from build123d import *
from build123d.topology import SkipClean

# Parameters (mm, degrees)
CROQUIS3_W                   = 38
CROQUIS3_H                   = 38
SALIENTE_EXTRUIR9_DEPTH      = 1
SALIENTE_EXTRUIR10_START     = -11
SALIENTE_EXTRUIR10_OUTLINE_W = 38
SALIENTE_EXTRUIR10_OUTLINE_H = 38
SALIENTE_EXTRUIR10_DEPTH     = 10
CROQUIS13_W                  = 38
CROQUIS13_H                  = 38
SALIENTE_EXTRUIR15_DEPTH     = 3
CROQUIS14_R                  = 1.5
CORTAR_EXTRUIR1_DEPTH        = 14
CROQUIS15_W                  = 38
CROQUIS15_H                  = 24.129942315
CROQUIS15_R                  = 1.5
CROQUIS15_R_2                = 3.5
SALIENTE_EXTRUIR16_DEPTH     = 1
CORTAR_EXTRUIR2_DEPTH        = 14
CROQUIS17_R                  = 1.5
SALIENTE_EXTRUIR17_DEPTH     = 5
CROQUIS18_R                  = 1.5
CROQUIS18_W                  = 12
CROQUIS18_H                  = 12
SALIENTE_EXTRUIR18_DEPTH     = 5
CORTAR_EXTRUIR3_DEPTH        = 3
CROQUIS20_R                  = 3
CROQUIS20_R_2                = 1.5
SALIENTE_EXTRUIR19_DEPTH     = 3
REDONDEO11_R                 = 1
CROQUIS21_W                  = 12
CROQUIS21_H                  = 3
SALIENTE_EXTRUIR20_DEPTH     = 10


# Read off the part's stored shape, not the designer's step: Saliente-Extruir10
with BuildPart() as part:
    # Croquis3 → Saliente-Extruir9 (new body)
    with BuildSketch(Plane.XY.offset(5)):
        Polygon((19, -5.370057685), (26.870057685, 2.5), (26.870057685, 40.5), (19, 48.370057685), (-19, 48.370057685), (-26.870057685, 40.5), (-26.870057685, 2.5), (-19, -5.370057685), align=None)
        with Locations((0, 21.5)):
            Rectangle(CROQUIS3_W, CROQUIS3_H, mode=Mode.SUBTRACT)
    extrude(amount=-SALIENTE_EXTRUIR9_DEPTH)

    # Saliente-Extruir10 outline → Saliente-Extruir10 (add)
    with BuildSketch(Plane(origin=(0, 0, 4), x_dir=(-1, 0, 0), z_dir=(0, 0, -1)).offset(SALIENTE_EXTRUIR10_START)):
        Polygon((-26.870057685, 2.5), (-19, -5.370057685), (19, -5.370057685), (26.870057685, 2.5), (26.870057685, 40.5), (19, 48.370057685), (-19, 48.370057685), (-26.870057685, 40.5), align=None)
        with Locations((0, 21.5)):
            Rectangle(SALIENTE_EXTRUIR10_OUTLINE_W, SALIENTE_EXTRUIR10_OUTLINE_H, mode=Mode.SUBTRACT)
    extrude(amount=SALIENTE_EXTRUIR10_DEPTH)

    # Croquis13 → Saliente-Extruir15 (add)
    with BuildSketch(Plane.XY.offset(15)):
        with BuildLine():
            Line((-22.5, 44.870057685), (-22.5, -1))
            Line((-22.5, -1), (22.5, -1))
            Line((22.5, -1), (22.5, 44.870057685))
            Line((22.5, 44.870057685), (19.292893219, 48.077164466))
            ThreePointArc((19.292893219, 48.077164466), (18.96846987, 48.293937218), (18.585786438, 48.370057685))
            Line((18.585786438, 48.370057685), (-18.585786438, 48.370057685))
            ThreePointArc((-18.585786438, 48.370057685), (-18.96846987, 48.293937218), (-19.292893219, 48.077164466))
            Line((-19.292893219, 48.077164466), (-22.5, 44.870057685))
        make_face()
        with Locations((0, 21.5)):
            Rectangle(CROQUIS13_W, CROQUIS13_H, mode=Mode.SUBTRACT)
    extrude(amount=SALIENTE_EXTRUIR15_DEPTH)

    # Croquis14 → Cortar-Extruir1 (cut)
    with BuildSketch(Plane(origin=(0, 0, 4), x_dir=(-1, 0, 0), z_dir=(0, 0, -1))):
        with Locations((10, 44.97415474)):
            Circle(CROQUIS14_R)
        with Locations(Location((-10, 44.97415474, 0), (0, 0, 180))):
            Circle(CROQUIS14_R)
    extrude(amount=-CORTAR_EXTRUIR1_DEPTH, mode=Mode.SUBTRACT)

    # Croquis15 → Saliente-Extruir16 (add)
    with BuildSketch(Plane(origin=(0, 0, 4), x_dir=(-1, 0, 0), z_dir=(0, 0, -1))):
        with Locations((0, 28.435028843)):
            Rectangle(CROQUIS15_W, CROQUIS15_H)
        with Locations((0, 34.97415474)):
            Circle(CROQUIS15_R, mode=Mode.SUBTRACT)
        with Locations((0, 25.370057685)):
            Circle(CROQUIS15_R_2, mode=Mode.SUBTRACT)
    extrude(amount=-SALIENTE_EXTRUIR16_DEPTH)

    # Croquis16 → Cortar-Extruir2 (cut)
    with BuildSketch(Plane(origin=(0, 0, 4), x_dir=(-1, 0, 0), z_dir=(0, 0, -1))):
        Polygon((-19, 2.5), (-19, 16.370057685), (-26.870057685, 24.24011537), (-26.870057685, 2.5), (-19, -5.370057685), (19, -5.370057685), (26.870057685, 2.5), (26.870057685, 24.24011537), (19, 16.370057685), (19, 2.5), align=None)
    extrude(amount=-CORTAR_EXTRUIR2_DEPTH, mode=Mode.SUBTRACT)

    # Croquis17 → Saliente-Extruir17 (add)
    with SkipClean():  # the faces are left unmerged after this step: merging them gives an invalid solid
        with BuildSketch(Plane.XY.offset(5)):
            Polygon((6, 31.370057685), (6, 25.370057685), (6, 19.370057685), (6, 16.370057685), (19, 16.370057685), (19, 40.5), (-19, 40.5), (-19, 16.370057685), (-6, 16.370057685), (-6, 19.370057685), (-6, 31.370057685), align=None)
            with Locations((0, 34.97415474)):
                Circle(CROQUIS17_R, mode=Mode.SUBTRACT)
        extrude(amount=SALIENTE_EXTRUIR17_DEPTH)
    add(part.part.scale(1), mode=Mode.REPLACE)  # the faces are merged on a copy

    # Croquis18 → Saliente-Extruir18 (add)
    # profile 1 of 2: a face of its own
    with BuildSketch(Plane.XY.offset(10)):
        Polygon((-6, 31.370057685), (6, 31.370057685), (6, 16.370057685), (19, 16.370057685), (19, 40.5), (-19, 40.5), (-19, 16.370057685), (-6, 16.370057685), align=None)
        with Locations(Location((0, 34.97415474, 0), (0, 0, 180))):
            Circle(CROQUIS18_R, mode=Mode.SUBTRACT)
    # profile 2 of 2: a face of its own
    with BuildSketch(Plane.XY.offset(10)):
        with Locations((0, 25.370057685)):
            Rectangle(CROQUIS18_W, CROQUIS18_H)
    extrude(amount=SALIENTE_EXTRUIR18_DEPTH)

    # Croquis19 → Cortar-Extruir3 (cut)
    with BuildSketch(Plane.XY.offset(18)):
        Polygon((-22.5, 19.870057685), (-19, 16.370057685), (-19, 21.370057685), (-22.5, 21.370057685), align=None)
        Polygon((19, 16.370057685), (22.5, 19.870057685), (22.5, 21.370057685), (19, 21.370057685), align=None)
    extrude(amount=-CORTAR_EXTRUIR3_DEPTH, mode=Mode.SUBTRACT)

    # Croquis20 → Saliente-Extruir19 (add)
    with BuildSketch(Plane.XY.offset(15)):
        with Locations(Location((0, 34.97415474, 0), (0, 0, 180))):
            Circle(CROQUIS20_R)
        with Locations(Location((0, 34.97415474, 0), (0, 0, 180))):
            Circle(CROQUIS20_R_2, mode=Mode.SUBTRACT)
    extrude(amount=SALIENTE_EXTRUIR19_DEPTH)

    # Redondeo11
    redondeo11_edges = [part.edges().sort_by_distance(p)[0] for p in [
        (26.870057685, 40.5, 10),
        (19, 48.370057685, 10),
        (-19, 48.370057685, 10),
        (-26.870057685, 40.5, 10),
        (26.870057685, 24.24011537, 9.5),
        (19, 16.370057685, 9.5),
        (-26.870057685, 24.24011537, 9.5),
        (-19, 16.370057685, 9.5),
    ]]
    fillet(redondeo11_edges, radius=REDONDEO11_R)

    # Croquis21 → Saliente-Extruir20 (add)
    with BuildSketch(Plane.XY.offset(5)):
        with Locations((0, 17.870057685)):
            Rectangle(CROQUIS21_W, CROQUIS21_H)
    extrude(amount=SALIENTE_EXTRUIR20_DEPTH)


solid = part.part
Design review of the part built by this model. Coordinates are the model's own, in mm. A direction names the side the tool comes from. Give positions to 0.01 mm unless a question says otherwise; leave off trailing zeros. Order: outer loops, then holes, each group sorted by start corner. A loop starts at its lowest first (then second) coordinate and runs counter-clockwise, first axis right, second up.
1. Add section A-A, the plane z = 17.25. State the section outline as (x, y) points, then the cut area to 3 significant figures.
Solution:
outline: (-22.5, 21.37) - (-19, 21.37) - (-19, 40.5) - (19, 40.5) - (19, 21.37) - (22.5, 21.37) - (22.5, 44.87) - (19.29, 48.08) arc R1 ccw to (18.59, 48.37) - (-18.59, 48.37) arc R1 ccw to (-19.29, 48.08) - (-22.5, 44.87) - close; circle Ø6 at (0, 34.97); hole circle Ø3 at (-10, 44.97); hole circle Ø3 at (0, 34.97); hole circle Ø3 at (10, 44.97)
area: 483 mm2
2. To check wall thickness, follow L1, parallel to Y at x = 0, z = 4.65; L2, parallel to Y at x = -10, z = 8.25; L3, parallel to X at y = 25, z = 15.25. State the ranges of each line that lie inside material, in increasing order.
Solution:
L1: y = 16.37 to 21.87, 28.87 to 33.47, 36.47 to 48.37
L2: y = 16.37 to 43.47, 46.47 to 48.37
L3: x = -22.5 to -19, 19 to 22.5
3. For pin 1 Ø2.5 at (x, y) = (0, 34.97) entering from -Z; pin 2 Ø2.5 at (x, z) = (-21.5, 16) entering from -Y, all flat-tipped, find the tip position at first contact; note any pin that passes through.
Solution:
pin 1: passes through
pin 2: stops at y = 18.12
4. Mouldability with a two-part tool opening along Y and no side actions: class faces 6 (the flat face through (0, 31.37, 7)), 7 (the flat face through (-26.87, 32, 10)), 8 (the flat face through (-6, 25, 7)), 9 (the flat face through (0, 48.37, 11)) as +Y half, -Y half, draft (parallel to the pull), parting line (faces both ways), or undercut.
Solution:
face 6: undercut
face 7: draft
face 8: undercut
face 9: +Y half
5. Add section C-C, the plane z = 13. State the section outline as (x, y) points, then the cut area to 3 significant figures.
Solution:
outline: (-26.87, 24.65) arc R1 ccw to (-26.58, 23.95) - (-19.29, 16.66) arc R1 ccw to (-18.59, 16.37) - (18.59, 16.37) arc R1 ccw to (19.29, 16.66) - (26.58, 23.95) arc R1 ccw to (26.87, 24.65) - (26.87, 40.09) arc R1 ccw to (26.58, 40.79) - (19.29, 48.08) arc R1 ccw to (18.59, 48.37) - (-18.59, 48.37) arc R1 ccw to (-19.29, 48.08) - (-26.58, 40.79) arc R1 ccw to (-26.87, 40.09) - close; hole circle Ø3 at (-10, 44.97); hole circle Ø3 at (0, 34.97); hole circle Ø3 at (10, 44.97)
area: 1,570 mm2
6. Add section B-B, the plane x = -10. State the section outline as (y, z) points.
Solution:
outline: (16.37, 4) - (43.47, 4) - (43.47, 18) - (40.5, 18) - (40.5, 15) - (16.37, 15) - close; (46.47, 4) - (48.37, 4) - (48.37, 18) - (46.47, 18) - close
7. Add section D-D, the plane x = 0. State the section outline as (y, z) points, then the cut area to 3 significant figures.
Solution:
outline: (16.37, 4) - (21.87, 4) - (21.87, 5) - (19.37, 5) - (19.37, 10) - (31.37, 10) - (31.37, 5) - (28.87, 5) - (28.87, 4) - (33.47, 4) - (33.47, 18) - (31.97, 18) - (31.97, 15) - (16.37, 15) - close; (36.47, 4) - (48.37, 4) - (48.37, 18) - (40.5, 18) - (40.5, 15) - (37.97, 15) - (37.97, 18) - (36.47, 18) - close
area: 285 mm2
8. Tool access review of faces 1 (the flat face through (0, 25, 10)), 2 (the cylindrical face through (0.46, 28.84, 4.49)), 3 (the flat face through (19, 31, 16)), 4 (the flat face through (-22.5, 33, 16)), 5 (the flat face through (21, 21.37, 17)): name each direction out of +Z, -Z, +X, -X, +Y, -Y from which nothing blocks a thin tool from reaching the whole face with its end or side.
Solution:
face 1: none
face 2: -Z
face 3: +Z, -Y
face 4: +Z, -X, +Y, -Y
face 5: +Z, +X, -X, -Y
